```python
from build123d import *

# Parameters (mm, degrees)
SKETCH1_W           = 15
SKETCH1_H           = 7.5
BOSS_EXTRUDE1_DEPTH = 4
SKETCH3_W           = 15
SKETCH3_H           = 2.75
BOSS_EXTRUDE3_DEPTH = 15
CUT_EXTRUDE2_DEPTH  = 22.685248442
SKETCH6_R           = 2.75
CUT_EXTRUDE3_DEPTH  = 23.5
SKETCH10_R          = 8
CUT_EXTRUDE6_DEPTH  = 3
CUT_EXTRUDE9_START  = -1.75
SKETCH13_R          = 8
CUT_EXTRUDE9_DEPTH  = 1.75
CUT_EXTRUDE8_DEPTH  = 3
CUT_EXTRUDE10_DEPTH = 1.75


with BuildPart() as part:
    # Sketch1 → Boss-Extrude1 (new body)
    with BuildSketch(Plane(origin=(0, 0, 0), x_dir=(1, 0, 0), z_dir=(0, 1, 0))):
        with Locations((7.5, 3.75)):
            Rectangle(SKETCH1_W, SKETCH1_H)
    extrude(amount=BOSS_EXTRUDE1_DEPTH)

    # Sketch3 → Boss-Extrude3 (add)
    with BuildSketch(Plane.XZ):
        with Locations((7.5, -3.125)):
            Rectangle(SKETCH3_W, SKETCH3_H)
    extrude(amount=BOSS_EXTRUDE3_DEPTH)

    # Sketch5 → Cut-Extrude2 (cut, through all)
    with BuildSketch(Plane(origin=(0, 0, -4.5), x_dir=(-1, 0, 0), z_dir=(0, 0, -1))):
        with BuildLine():
            Line((-15, -7.5), (-15, -17.341994959))
            Line((-15, -17.341994959), (0, -17.341994959))
            Line((0, -17.341994959), (0, -7.5))
            ThreePointArc((0, -7.5), (-7.5, -15), (-15, -7.5))
        make_face()
    extrude(amount=-CUT_EXTRUDE2_DEPTH, mode=Mode.SUBTRACT)

    # Sketch6 → Cut-Extrude3 (cut, through all)
    with BuildSketch(Plane(origin=(0, 0, -7.5), x_dir=(-1, 0, 0), z_dir=(0, 0, -1))):
        with Locations((-7.5, -7.5)):
            Circle(SKETCH6_R)
    extrude(amount=-CUT_EXTRUDE3_DEPTH, mode=Mode.SUBTRACT)

    # Sketch10 → Cut-Extrude6 (cut)
    with BuildSketch(Plane(origin=(0, 0, -7.5), x_dir=(-1, 0, 0), z_dir=(0, 0, -1))):
        with Locations((-7.5, -7.5)):
            Circle(SKETCH10_R)
    extrude(amount=-CUT_EXTRUDE6_DEPTH, mode=Mode.SUBTRACT)

    # Sketch13 → Cut-Extrude9 (cut)
    with BuildSketch(Plane.XY.offset(CUT_EXTRUDE9_START)):
        with Locations((7.5, -7.5)):
            Circle(SKETCH13_R)
    extrude(amount=CUT_EXTRUDE9_DEPTH, mode=Mode.SUBTRACT)

    # Sketch12 → Cut-Extrude8 (cut)
    with BuildSketch(Plane(origin=(0, 0, -7.5), x_dir=(-1, 0, 0), z_dir=(0, 0, -1))):
        Polygon((-10.283882181, 0), (-15, 1), (-15, 0), align=None)
        Polygon((-4.716117819, 0), (0, 1), (0, 0), align=None)
    extrude(amount=-CUT_EXTRUDE8_DEPTH, mode=Mode.SUBTRACT)

    # Sketch14 → Cut-Extrude10 (cut)
    with BuildSketch(Plane.XY):
        Polygon((4.716117819, 0), (0, 1), (0, 0), align=None)
        Polygon((10.283882181, 0), (15, 1), (15, 0), align=None)
    extrude(amount=-CUT_EXTRUDE10_DEPTH, mode=Mode.SUBTRACT)

    # Mirror1: part across plane


with BuildPart() as part_1:
    add(part.part)
    add(part.part.mirror(Plane(origin=(0, 4, 0), x_dir=(1, 0, 0), z_dir=(0, 0, -1))))


solid = part_1.part
```
Model file for the job. Use its own axes, mm. A direction names the side the tool comes from. Give positions to 0.01 mm unless a question says otherwise; leave off trailing zeros. Loops run counter-clockwise (first coordinate to the right, second up) from the corner with the lowest first, then second, coordinate; pieces in that order, holes last. Notation, with made-up numbers: (73.5, 55) -> (79.5, 55) arc R24 ccw to (79.5, 68) -> close; hole circle Ø3 at (28.25, -10.75). An arc over 180 degrees is marked (long way). Write each question's results on one line, items separated by ' | '.
(1) Cut at A-A on x = 7.5. List the corners of the cut face in (y, z), and give its area (4 significant figures).
Geometry results:
outline: (-15, -4.5) -> (-10.25, -4.5) -> (-10.25, -1.75) -> (-15, -1.75) -> close; (-15, 1.75) -> (-10.25, 1.75) -> (-10.25, 4.5) -> (-15, 4.5) -> close; (-4.75, -4.5) -> (0.5, -4.5) -> (0.5, -7.5) -> (4, -7.5) -> (4, 7.5) -> (0.5, 7.5) -> (0.5, 4.5) -> (-4.75, 4.5) -> (-4.75, 1.75) -> (0.5, 1.75) -> (0.5, -1.75) -> (-4.75, -1.75) -> close | area: 107.5 mm²
(2) Probe line 1 along Y through (x, z) = (7.5, 2.75); line 2 along Z through (x, y) = (11.75, 0); line 3 along X through (y, z) = (-7.75, 3). List the from-to ranges inside material, lowest first.
Geometry results:
line 1: y = -15 to -10.25, -4.75 to 4 | line 2: z = -4.5 to -1.75, 1.75 to 4.5 | line 3: x = 0 to 4.76, 10.24 to 15
(3) Tool access for faces 4 (the flat face through (2.391, 0.493, -0.024)), 5 (the flat face through (12.609, 0.493, -0.024)), 6 (the cylindrical face through (7.5, 0.5, 6)), 7 (the cylindrical face through (7.5, 0.5, -6)): list every direction of +Z, -Z, +X, -X, +Y, -Y with a clear straight run to the whole face (end or side of a thin tool).
Geometry results:
face 4: -X, -Y | face 5: +X, -Y | face 6: +Z, -Y | face 7: -Z, -Y
(4) Cut at D-D on y = -11. List the corners of the cut face in (x, z), and give its area (3 significant figures).
Geometry results:
outline: (0.87, -4.5) -> (14.13, -4.5) -> (14.13, -1.75) -> (0.87, -1.75) -> close; (0.87, 1.75) -> (14.13, 1.75) -> (14.13, 4.5) -> (0.87, 4.5) -> close | area: 73.0 mm²
(5) Flat gauge pins, fed straight in: pin 1 Ø1.5 at (x, y) = (10.5, -7) entering from -Z; pin 2 Ø4.5 at (x, y) = (4.5, -3.5) entering from +Z; pin 3 Ø5 at (x, y) = (7.5, -7.5) entering from +Z; pin 4 Ø2 at (x, z) = (2, 3.5) entering from -Y. Where does each tip first touch, or does it go through?
Geometry results:
pin 1: stops at z = -4.5 | pin 2: stops at z = 4.5 | pin 3: passes through | pin 4: stops at y = -13.5
(6) Cut at C-C on z = 4.25. List the corners of the cut face in (x, y), and give its area (3 significant figures).
Geometry results:
outline: (0, -7.5) arc R7.5 ccw to (15, -7.5) -> (15, 4) -> (0, 4) -> close; hole circle Ø5.5 at (7.5, -7.5) | area: 237 mm²
(7) Cut at B-B on y = -8.25. List the corners of the cut face in (x, z), and give its area (3 significant figures).
Geometry results:
outline: (0.04, -4.5) -> (4.85, -4.5) -> (4.85, -1.75) -> (0.04, -1.75) -> close; (0.04, 1.75) -> (4.85, 1.75) -> (4.85, 4.5) -> (0.04, 4.5) -> close; (10.15, -4.5) -> (14.96, -4.5) -> (14.96, -1.75) -> (10.15, -1.75) -> close; (10.15, 1.75) -> (14.96, 1.75) -> (14.96, 4.5) -> (10.15, 4.5) -> close | area: 53.0 mm²
(8) Pull direction X, two halves, no side cores. Call faces 1 (the flat face through (2.391, 0.493, 6.021)), 2 (the flat face through (12.609, 0.493, 6.021)), 3 (the cylindrical face through (7.5, 0.5, 0)): released by +X, released by -X, zero draft, split by the parting line, or undercut.
Geometry results:
face 1: released by -X | face 2: released by +X | face 3: undercut
